Model file for the job. Use its own axes, mm. A direction names the side the tool comes from. Give positions to 0.01 mm unless a question says otherwise; leave off trailing zeros. Write each loop counter-clockwise with the first axis right and the second up, starting at its lowest first coordinate (ties: lowest second). Pieces come first, ordered by that corner, then holes. Notation, with made-up numbers: (-19.75, 1.25) - (19.25, 1.25) arc R28 cw to (19.25, 27.25) - close; hole circle Ø10 at (77.5, 22.5). An arc over 180 degrees is marked (long way). Use CSV: the item, a comma, the result in double quotes.
from build123d import *

# Parameters (mm, degrees)
F1_DEPTH = 317.5
F2_T     = -3.175
F4_DEPTH = 1.5875
F5_W     = 508
F5_H     = 863.6
F6_DEPTH = 4.4911280605


with BuildPart() as f1:
    # F0 (on Right) → F1 (new body, symmetric)
    with BuildSketch(Plane.YZ):
        Polygon((-340.995, 340.995), (0, 0), (0, 1774.19), (-340.995, 1433.195), align=None)
    extrude(amount=F1_DEPTH, both=True)

    # F2
    f2_openings = [f1.faces().sort_by_distance(p)[0] for p in [
        (0, 0, 887.095),
    ]]
    offset(amount=F2_T, openings=f2_openings)

    # F3 (on Front) → F4 (join, symmetric)
    with BuildSketch(Plane.XZ):
        Polygon((-273.1135, 247.904), (273.1135, 247.904), (273.1135, 0), (317.5, 0), (317.5, 247.904), (317.5, 1526.286), (317.5, 1774.19), (273.1135, 1774.19), (273.1135, 1526.286), (-273.1135, 1526.286), (-273.1135, 1774.19), (-317.5, 1774.19), (-317.5, 1526.286), (-317.5, 247.904), (-317.5, 0), (-273.1135, 0), align=None)
    extrude(amount=F4_DEPTH, both=True)

    # F5 (on face) → F6 (cut, through all)
    with BuildSketch(Plane.XZ.offset(340.995)):
        with Locations((0, 1001.395)):
            Rectangle(F5_W, F5_H)
    extrude(amount=-F6_DEPTH, mode=Mode.SUBTRACT)


solid = f1.part
(1) Wall check: probe 1 along X at (y, z) = (-110.5, 283) (3 decimals); probe 2 along Y at (x, z) = (268, 540) (1 decimal); probe 3 along Y at (x, z) = (-45, 1021.5). Give the ranges that are in metal, low to high. Write a range as [from, to].
Checked values:
probe 1,"x = [-317.5, -314.325], [314.325, 317.5]"
probe 2,"y = [-341, -337.8], [-1.6, 1.6]"
probe 3,"y = [-1.59, 1.59]"
(2) Saw through at D-D, the plane y = -57. List the corners of the cut face in (x, z) (3 decimals), then the cut area to 3 significant figures.
Checked values:
outline,"(-317.5, 57) - (317.5, 57) - (317.5, 1717.19) - (-317.5, 1717.19) - close; hole (-314.325, 61.49) - (314.325, 61.49) - (314.325, 1712.7) - (-314.325, 1712.7) - close"
area,"16,200 mm^2"
(3) Saw through at C-C, the plane z = 854. List the corners of the cut face in (x, y) (1 decimal).
Checked values:
outline,"(-317.5, -341) - (-254, -341) - (-254, -337.8) - (-314.3, -337.8) - (-314.3, -1.6) - (314.3, -1.6) - (314.3, -337.8) - (254, -337.8) - (254, -341) - (317.5, -341) - (317.5, 1.6) - (-317.5, 1.6) - close"
(4) Saw through at B-B, the plane y = -151.5. List the corners of the cut face in (x, z) (3 decimals).
Checked values:
outline,"(-317.5, 151.5) - (317.5, 151.5) - (317.5, 1622.69) - (-317.5, 1622.69) - close; hole (-314.325, 155.99) - (314.325, 155.99) - (314.325, 1618.2) - (-314.325, 1618.2) - close"
(5) 3-axis set-ups, long thin cutter, end or side, ignore diameter. For faces 1 (the face through (4.4, -171.27, 175.76)), 2 (the face through (-4, 1.588, 900)): which of +Z, -Z, +X, -X, +Y, -Y reach the whole face in a straight line?
Checked values:
face 1,"none"
face 2,"+Z, -Z, +X, -X, +Y"
(6) Flat gauge pins, fed straight in: P1, Ø10, axis at x = 140.5, y = -85, coming from the +Z side; P2, Ø2, axis at x = 240, y = -303, coming from the +Z side; P3, Ø3.5, axis at x = 40, y = -339, coming from the +Z side. Where does each tip first touch, or does it go through?
Checked values:
P1,"stops at z = 1694.19"
P2,"stops at z = 1472.19"
P3,"stops at z = 1436.94"
(7) Pull direction Z, two halves, no side cores. Call faces 3 (the face through (4.4, -166.5, 1603.2)), 4 (the face through (4, -340.995, 531)), 5 (the face through (4, -173, 173)): released by +Z, released by -Z, zero draft, split by the parting line, or undercut.
Checked values:
face 3,"undercut"
face 4,"zero draft"
face 5,"released by -Z"
(8) Saw through at A-A, the plane x = -58.5. List the corners of the cut face in (y, z) (1 decimal).
Checked values:
outline,"(-341, 341) - (0, 0) - (0, 4.5) - (-337.8, 342.3) - (-337.8, 569.6) - (-341, 569.6) - close; (-341, 1433.2) - (-336.5, 1433.2) - (0, 1769.7) - (0, 1774.2) - close; (-1.6, 247.9) - (1.6, 247.9) - (1.6, 1526.3) - (-1.6, 1526.3) - close"
